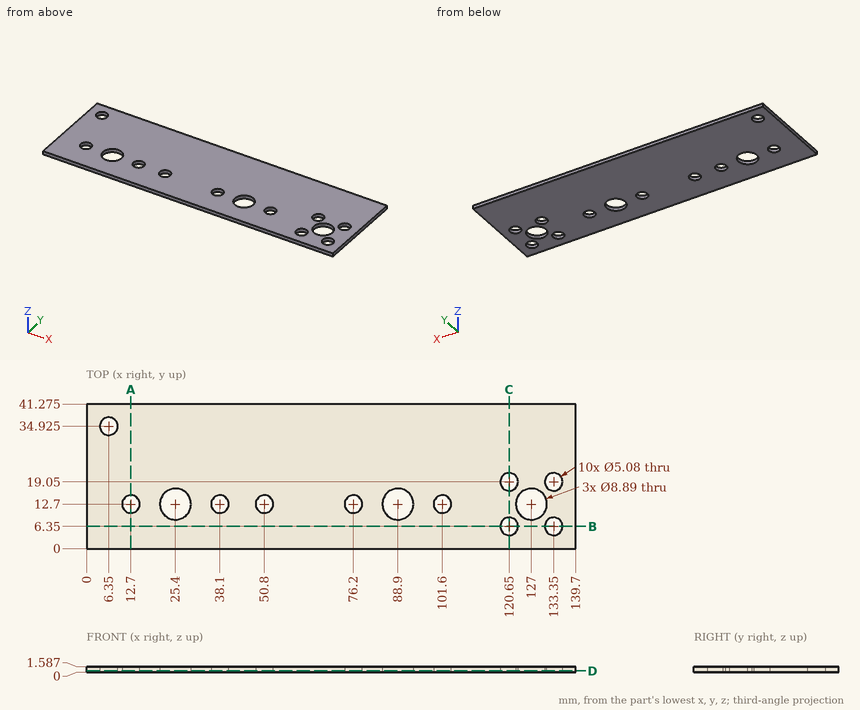
Here's the drawing with two shaded views (mm, measured from the low corner). I have some questions. Round coordinates to 2 decimals unless told otherwise and drop trailing zeros. Loops run counter-clockwise (first coordinate to the right, second up) from the corner with the lowest first, then second, coordinate; pieces in that order, holes last. Notation, with made-up numbers: (54.25, 24.25) -> (78.25, 24.25) arc R10 cw to (78.25, 33.25) -> close; hole circle Ø2 at (33, -23). An arc over 180 degrees is marked (long way). Answer as CSV lines item,"result". Start each with the question number.
1. Imagine slicing it at D-D on z = 0.35. State how many separate pieces and enclosed holes the cut face has, plus the area to 3 significant figures.
2. I need wall thicknesses on probe 1 along Y at (x, z) = (120.65, 1.05) (1 decimal); probe 2 along X at (y, z) = (6, 1.25) (1 decimal); probe 3 along Y at (x, z) = (38.1, 0.9) (1 decimal). Which ranges of each line are inside material? Lowest first, please. Write a range as from..to.
3. Imagine slicing it at A-A on x = 12.7. Write out the boundary of the cut face in (y, z) (1 decimal).
4. Imagine slicing it at B-B on y = 6.35. Write out the boundary of the cut face in (x, z).
5. I'm going to push a flat-ended pin straight in: P1, Ø4, axis at x = 12.7, y = 12.7, coming from the +Z side. Where does the tip first touch, or does it pass through?
6. Imagine slicing it at C-C on x = 120.65. Write out the boundary of the cut face in (y, z) (1 decimal).
Solution:
1,separate pieces,"1"
1,enclosed holes,"13"
1,area,"5,380 mm²"
2,probe 1,"0..3.8, 8.9..16.5, 21.6..41.3"
2,probe 2,"0..118.1, 123.2..130.8, 135.9..139.7"
2,probe 3,"0..10.2, 15.2..41.3"
3,outline,"(0, 0) -> (10.2, 0) -> (10.2, 1.6) -> (0, 1.6) -> close; (15.2, 0) -> (41.3, 0) -> (41.3, 1.6) -> (15.2, 1.6) -> close"
4,outline,"(0, 0) -> (118.11, 0) -> (118.11, 1.59) -> (0, 1.59) -> close; (123.19, 0) -> (130.81, 0) -> (130.81, 1.59) -> (123.19, 1.59) -> close; (135.89, 0) -> (139.7, 0) -> (139.7, 1.59) -> (135.89, 1.59) -> close"
5,P1,"through"
6,outline,"(0, 0) -> (3.8, 0) -> (3.8, 1.6) -> (0, 1.6) -> close; (8.9, 0) -> (16.5, 0) -> (16.5, 1.6) -> (8.9, 1.6) -> close; (21.6, 0) -> (41.3, 0) -> (41.3, 1.6) -> (21.6, 1.6) -> close"
